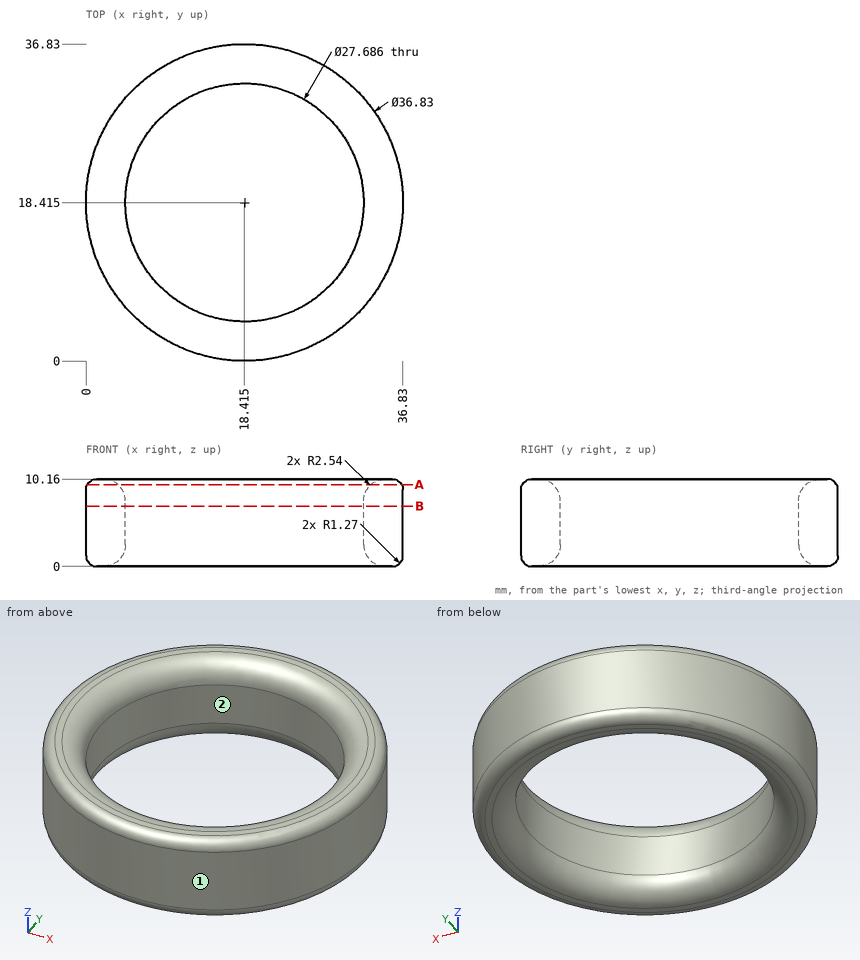
Source: three-view drawing plus pictorial views. Frame: mm from the lowest corner of the part. Give positions to 0.01 mm unless a question says otherwise; leave off trailing zeros. Write each loop counter-clockwise with the first axis right and the second up, starting at its lowest first coordinate (ties: lowest second). Pieces come first, ordered by that corner, then holes. Notation, with made-up numbers: (-15.5, 7) - (-4.5, 7) arc R27 cw to (-4.5, 28) - close; hole circle Ø7 at (-3, -39). An arc over 180 degrees is marked (long way). Write item = value, one per line. Start each with the question number.
1. Section query B-B, the plane z = 7. Output: boundary loops of the cut face in (x, y) (3 decimals), then the cut area to 3 significant figures.
2. Mould query, pull axis Y, two halves, no side actions, for the marked faces 1 and 2. Classes: released by +Y, released by -Y, zero draft, split by the parting line, or undercut.
3. First-contact query: pin 1 Ø3 at (y, z) = (25, 9) entering from -X; pin 2 Ø22 at (x, y) = (18.415, 18.415) entering from -Z; pin 3 Ø1.5 at (x, z) = (6.5, 2) entering from -Y; pin 4 Ø4 at (y, z) = (7, 4.5) entering from -X. Flat tips, straight axial feed; report the tip coordinate or a pass-through.
4. Section query A-A, the plane z = 9.5. Output: boundary loops of the cut face in (x, y) (3 decimals).
5. Ray query, L1, parallel to Y at x = 8, z = 3.75; L2, parallel to Y at x = 27, z = 8.75; L3, parallel to X at y = 22, z = 3. Return the intervals inside material, ascending.
Check sheet entries:
q1.outline = circle Ø36.83 at (18.415, 18.415); hole circle Ø27.686 at (18.415, 18.415)
q1.area = 463 mm2
q2.face_1 = split by the parting line
q2.face_2 = undercut
q3.pin_1 = 0.72
q3.pin_2 = through
q3.pin_3 = 3.77
q3.pin_4 = 2.59
q4.outline = circle Ø36.518 at (18.415, 18.415); hole circle Ø29.35 at (18.415, 18.415)
q5.L1 = 3.23 to 9.3, 27.53 to 33.6
q5.L2 = 2.12 to 7.22, 29.61 to 34.71
q5.L3 = 0.35 to 5.04, 31.79 to 36.48
